Read the model definition and answer for the solid it produces. Units are mm, in the model's axes. A direction names the side the tool comes from. Coordinates: 2 decimals unless noted, no trailing zeros. Write each loop counter-clockwise with the first axis right and the second up, starting at its lowest first coordinate (ties: lowest second). Pieces come first, ordered by that corner, then holes.
(1) Which of the six approach directions +Z, -Z, +X, -X, +Y, -Y give full straight-line access (tool end or side, diameter ignored) to faces 1 (the flat face through (0, -5, -15)), 2 (the flat face through (-7.5, 0, -15)), 3 (the flat face through (-16, 0, 2.16)), 4 (the flat face through (0, 5, -15))?
(2) The part is cut by section D-D, the plane x = 10. Determine the outline of the cut face in (y, z) (3 decimals), and give its area (3 significant figures).
(3) The part is cut by section C-C, the plane z = -12.5. Determine the outline of the cut face in (x, y), and give its area (3 significant figures).
(4) The part is cut by section A-A, the plane x = 0. Determine the outline of the cut face in (y, z) (3 decimals), and give its area (3 significant figures).
(5) Determine the mould class of faces 5 (the flat face through (0, 0, 22.99)), 6 (the cylindrical face through (-15.61, -0.69, 12.43)), 7 (the cylindrical face through (13.582, -13.482, 1.065)) for opening direction X: pulls with the +X half, pulls with the -X half, needs draft (parallel to the pull), parting line crosses it, or undercut.
(6) The part is cut by section B-B, the plane y = 0. Determine the outline of the cut face in (x, z) (3 decimals).
(7) Given pin 1 (4.5 mm diameter, centred on y = -1, z = -14, fed in from -X); pin 2 (1 mm diameter, centred on y = -6, z = 15.5, fed in from +X) (3 decimals); pin 3 (8 mm diameter, centred on x = -4.5, y = -11.5, fed in from -Z); pin 4 (1.9 mm diameter, centred on x = -14.68, y = 14.68, fed in from -Z), each flat-ended and moving along its own axis, determine where each tip first touches the part or whether it passes through.
(8) Straight lines are drawn through the part: line 1 along Y through (x, z) = (14.68, 1.45) (3 decimals); line 2 along Z through (x, y) = (14.5, 5). For each, find the intervals that lie inside material, in ascending order.
Autodesk Inventor part; units mm, degrees
ref_plane "YZ Plane" through (0, 0, 0) normal (1, 0, 0) x (0, 1, 0)
ref_plane "XZ Plane" through (0, 0, 0) normal (0, 1, 0) x (-1, 0, 0)
ref_plane "XY Plane" through (0, 0, 0) normal (0, 0, 1) x (1, 0, 0)
sketch "Sketch1" plane through (0, 0, 0) normal (0, 0, 1) x (1, 0, 0)
  line L0 (-18.265, 18.265) -> (18.265, 18.265)
  line L1 (18.265, 18.265) -> (18.265, -18.265)
  line L2 (18.265, -18.265) -> (-18.265, -18.265)
  line L3 (-18.265, -18.265) -> (-18.265, 18.265)
  point P0 (0, 0)
  point P1 (0, 18.265)
  point P2 (-18.265, 0)
  dimension "d0" = 36.53
  dimension "d1" = 36.53
extrude "Extrusion1" add sketch "Sketch1" along normal blind 2.16
chamfer "Chamfer1" distance 2 angle 45 4 edges at (18.265, 18.265, 1.08) (-18.265, 18.265, 1.08) (-18.265, -18.265, 1.08) (18.265, -18.265, 1.08)
sketch "Sketch2" plane through (0, 0, 2.16) normal (0, 0, 1) x (1, 0, 0)
  line L0 (-14.68, 14.68) -> (14.68, 14.68)
  line L1 (14.68, 14.68) -> (14.68, -14.68)
  line L2 (14.68, -14.68) -> (-14.68, -14.68)
  line L3 (-14.68, -14.68) -> (-14.68, 14.68)
  point P0 (0, 0)
  point P1 (0, 14.68)
  point P2 (-14.68, 0)
  dimension "d7" = 29.36
hole "Hole1" at (-14.68, 14.68, 2.16) at (14.68, 14.68, 2.16) at (-14.68, -14.68, 2.16) at (14.68, -14.68, 2.16) direction (0, 0, -1) diameter 3.25 end through all
sketch "Sketch3" plane through (0, 0, 2.16) normal (0, 0, 1) x (1, 0, 0)
  circle A0 centre (0, 0) radius 15.625
  dimension "d15" = 31.25
extrude "Extrusion2" add sketch "Sketch3" along normal blind 20.83
sketch "Sketch4" plane through (0, 0, 0) normal (0, 0, -1) x (-1, 0, 0)
  circle A0 centre (0, 0) radius 15
  dimension "d18" = 30
extrude "Extrusion3" add sketch "Sketch4" along normal blind 10.9
sketch "Sketch5" plane through (0, 0, -10.9) normal (0, 0, -1) x (-1, 0, 0)
  line L0 (-7.5, 5) -> (7.5, 5)
  line L1 (7.5, 5) -> (7.5, -5)
  line L2 (7.5, -5) -> (-7.5, -5)
  line L3 (-7.5, -5) -> (-7.5, 5)
  point P0 (0, 0)
  point P1 (0, 5)
  point P2 (7.5, 0)
  dimension "d21" = 15
  dimension "d22" = 10
extrude "Extrusion4" add sketch "Sketch5" along normal blind 9.21
properties part number "RJFTV21 X Amphenol Connector"
Computed:
1. face 1: -Z, +X, -X, -Y
1. face 2: -Z, -X, +Y, -Y
1. face 3: +Z
1. face 4: -Z, +X, -X, +Y
2. outline: (-18.265, 0) - (-11.18, 0) - (-11.18, -10.9) - (11.18, -10.9) - (11.18, 0) - (18.265, 0) - (18.265, 2.16) - (12.006, 2.16) - (12.006, 22.99) - (-12.006, 22.99) - (-12.006, 2.16) - (-18.265, 2.16) - close
2. area: 823 mm2
3. outline: (-7.5, -5) - (7.5, -5) - (7.5, 5) - (-7.5, 5) - close
3. area: 150 mm2
4. outline: (-18.265, 0) - (-15, 0) - (-15, -10.9) - (-5, -10.9) - (-5, -20.11) - (5, -20.11) - (5, -10.9) - (15, -10.9) - (15, 0) - (18.265, 0) - (18.265, 2.16) - (15.625, 2.16) - (15.625, 22.99) - (-15.625, 22.99) - (-15.625, 2.16) - (-18.265, 2.16) - close
4. area: 1,150 mm2
5. face 5: needs draft
5. face 6: parting line crosses it
5. face 7: undercut
6. outline: (-18.265, 0) - (-15, 0) - (-15, -10.9) - (-7.5, -10.9) - (-7.5, -20.11) - (7.5, -20.11) - (7.5, -10.9) - (15, -10.9) - (15, 0) - (18.265, 0) - (18.265, 2.16) - (15.625, 2.16) - (15.625, 22.99) - (-15.625, 22.99) - (-15.625, 2.16) - (-18.265, 2.16) - close
7. pin 1: stops at x = -7.5
7. pin 2: stops at x = 14.625
7. pin 3: stops at z = -10.9
7. pin 4: passes through
8. line 1: y = -18.265 to -16.305, -13.055 to 13.055, 16.305 to 18.265
8. line 2: z = 0 to 22.99
